For this review, use the dimensioned drawing (mm, ordinates from the lowest corner) and the shaded views. A direction names the side the tool comes from. Coordinates: 2 decimals unless noted, no trailing zeros. Loops run counter-clockwise (first coordinate to the right, second up) from the corner with the lowest first, then second, coordinate; pieces in that order, holes last. Notation, with made-up numbers: M 79.25,81.25 L 88.25,81.25 A12 cw 88.25,95.25 Z; hole C 33,42.25 d4. An arc over 180 degrees is marked long. One line per item, written item: value.
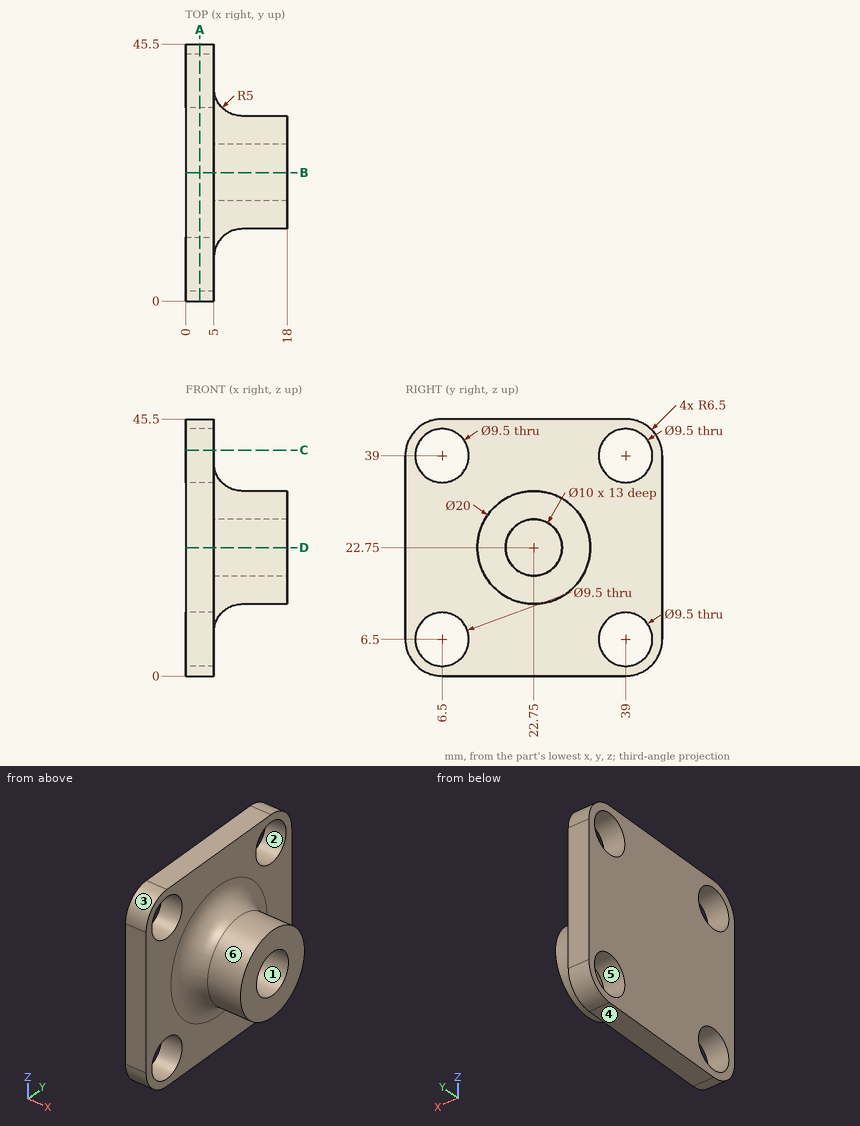
(1) Tool access review of the marked faces 1 and 2: name each direction out of +Z, -Z, +X, -X, +Y, -Y from which nothing blocks a thin tool from reaching the whole face with its end or side.
Checks:
face 1: +X
face 2: +X, -X
(2) To check wall thickness, follow L1, parallel to Z at x = 1.2, y = 39; L2, parallel to X at y = 2, z = 25; L3, parallel to Z at x = 2.75, y = 42. State the ranges of each line that lie inside material, in increasing order. Write a range as [from, to].
Checks:
L1: [0, 1.75], [11.25, 34.25], [43.75, 45.5]
L2: [0, 5]
L3: [0.73, 2.82], [10.18, 35.32], [42.68, 44.77]
(3) Draft analysis for pull direction Y (two halves, no side actions). For the marked faces 3, 4, 5 and 6, state which applies: pulls with the +Y half, pulls with the -Y half, needs draft (parallel to the pull), parting line crosses it, or undercut.
Checks:
face 3: pulls with the -Y half
face 4: needs draft
face 5: undercut
face 6: parting line crosses it
(4) Insertion check: pin 1 Ø5 at (y, z) = (20.5, 22) entering from +X; pin 2 Ø2 at (y, z) = (38, 16) entering from -X; pin 3 Ø2 at (y, z) = (25, 10) entering from +X; pin 4 Ø5 at (x, y) = (13, 19) entering from +Z. Each pin has a flat end and moves straight along its axis. Give the tip position at first contact, or say it passes through.
Checks:
pin 1: x = 5
pin 2: x = 0
pin 3: x = 6.04
pin 4: z = 32.67
(5) Add section C-C on z = 40. State the section outline as (x, y) points, then the cut area to 3 significant figures.
Checks:
outline: M 0,0.08 L 5,0.08 L 5,1.86 L 0,1.86 Z; M 0,11.14 L 5,11.14 L 5,34.36 L 0,34.36 Z; M 0,43.64 L 5,43.64 L 5,45.42 L 0,45.42 Z
area: 134 mm^2
(6) Add section A-A on x = 2.5. State the section outline as (y, z) points.
Checks:
outline: M 0,6.5 A6.5 ccw 6.5,0 L 39,0 A6.5 ccw 45.5,6.5 L 45.5,39 A6.5 ccw 39,45.5 L 6.5,45.5 A6.5 ccw 0,39 Z; hole C 6.5,6.5 d9.5; hole C 6.5,39 d9.5; hole C 39,6.5 d9.5; hole C 39,39 d9.5
(7) Add section B-B on y = 22.75. State the section outline as (x, z) points.
Checks:
outline: M 0,0 L 5,0 L 5,7.75 A5 cw 10,12.75 L 18,12.75 L 18,17.75 L 5,17.75 L 5,27.75 L 18,27.75 L 18,32.75 L 10,32.75 A5 cw 5,37.75 L 5,45.5 L 0,45.5 Z
